from build123d import *

# Parameters (mm, degrees)
F3_DEPTH        = 1.651
F3_COPIES_COUNT = 10
F6_W            = 25.4
F6_H            = 5.08
F7_DEPTH        = 6.35
F8_R            = 1.5875
F9_DEPTH        = 3.81
F9_DEPTH_BACK   = 19.05
F10_R           = 9.906
F11_DEPTH       = 12.7
F12_R           = 9.525
F13_DEPTH       = 57.15
F14_R           = 7.62
F15_DEPTH       = 44.45


# Not quite as in the source:
# - a feature of the source that left no trace in its solid (it failed there, or was rolled back) is left out
# - a pattern or mirror of a feature is missing from the dataset's text; its kind, count and spacing are read off the source's solid


with BuildPart() as f1:
    # F0 (on Front) → F1 (revolve)
    with BuildSketch(Plane.XZ):
        with BuildLine():
            Line((-43.18, 1.016), (-45.6726494673, 1.016))
            ThreePointArc((-45.6726494673, 1.016), (-44.3886326409, 15.9499637645), (-57.15, 23.8125))
            Line((-57.15, 23.8125), (-57.15, -0.0228488987))
            Line((-57.15, -0.0228488987), (-43.18, -0.0228488987))
            Line((-43.18, -0.0228488987), (-43.18, 1.016))
        make_face()
    revolve(axis=Axis((-57.15, 0, 11.8948255506), (0, 0, 1)))

    # F2 (on face) → F3 (join)
    with BuildSketch(Plane.XY.offset(1.016)):
        with BuildLine():
            ThreePointArc((-45.6726494673, 0), (-45.6729398633, -0.081644771), (-45.6738110366, -0.1632854104))
            Line((-45.6738110366, -0.1632854104), (-43.1842536235, -0.1632854104))
            Line((-43.1842536235, -0.1632854104), (-43.1842536235, 0.3447145896))
            Line((-43.1842536235, 0.3447145896), (-45.6738110366, 0.3447145896))
            Line((-45.6738110366, 0.3447145896), (-45.6738110366, 0.1632854104))
            ThreePointArc((-45.6738110366, 0.1632854104), (-45.6729398633, 0.081644771), (-45.6726494673, 0))
        make_face()
    f3 = extrude(amount=F3_DEPTH)

    # F3_copies: F3 ×10 about axis
    f3_copies_axis = Axis((-57.15, 0, 0), (0, 0, 1))
    for i in range(1, F3_COPIES_COUNT):
        add(f3.rotate(f3_copies_axis, i * 360 / F3_COPIES_COUNT))

    # F6 (on offset) → F7 (cut)
    with BuildSketch(Plane.XY.offset(16.51)):
        with Locations((-57.15, 10.16)):
            Rectangle(F6_W, F6_H)
        with Locations((-57.15, -10.16)):
            Rectangle(F6_W, F6_H)
    extrude(amount=F7_DEPTH, mode=Mode.SUBTRACT)

    # F8 (on face) → F9 (cut, two sides)
    with BuildSketch(Plane.XZ.offset(7.62)) as f9_sk:
        with Locations((-57.15, 19.05)):
            Circle(F8_R)
    extrude(amount=F9_DEPTH, mode=Mode.SUBTRACT)
    extrude(f9_sk.sketch, amount=-F9_DEPTH_BACK, mode=Mode.SUBTRACT)

    # F10 (on face) → F11 (cut)
    with BuildSketch(Plane(origin=(0, 0, -0.0228488987), x_dir=(1, 0, 0), z_dir=(0, 0, -1))):
        with Locations((-57.15, 0)):
            Circle(F10_R)
    extrude(amount=-F11_DEPTH, mode=Mode.SUBTRACT)


with BuildPart() as f13:
    # F12 (on Top) → F13 (new body)
    with BuildSketch(Plane.XY):
        Circle(F12_R)
    extrude(amount=F13_DEPTH)

    # F14 (on face) → F15 (cut)
    with BuildSketch(Plane(origin=(0, 0, 0), x_dir=(1, 0, 0), z_dir=(0, 0, -1))):
        Circle(F14_R)
    extrude(amount=-F15_DEPTH, mode=Mode.SUBTRACT)


solid = f1.part
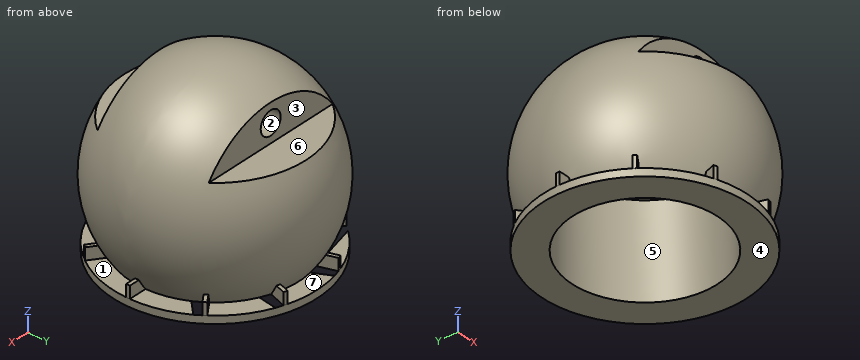
Input: part model. Units: mm. Frame: model coordinates. Face numbers are marked on the shaded views. A direction names the side the tool comes from. Give positions to 0.01 mm unless a question says otherwise; leave off trailing zeros. Write each loop counter-clockwise with the first axis right and the second up, starting at its lowest first coordinate (ties: lowest second). Pieces come first, ordered by that corner, then holes. Notation, with made-up numbers: M 11,-38 L 15,-38 A30 ccw 15,-12 Z; hole C -15.75,77 d9. An arc over 180 degrees is marked long. Use one line per item in the form item = value.
1. Cut plane B-B on x = -57.15. Return loops of the section in (y, z) (1 decimal).
Outcome:
outline = M -14,0 L -9.9,0 L -9.9,12.7 L 9.9,12.7 L 9.9,0 L 14,0 L 14,1 L 11.5,1 A14.3 ccw 12.5,16.5 L 7.6,16.5 L 7.6,17.5 L -7.6,17.5 L -7.6,16.5 L -12.5,16.5 A14.3 ccw -11.5,1 L -14,1 Z; M -7.6,20.6 L 7.6,20.6 L 7.6,21.6 A14.3 ccw -7.6,21.6 Z
2. First-contact query: P1, Ø2, axis at x = -54, y = -5.5, coming from the -Z side; P2, Ø0.7, axis at x = -53, y = -12.5, coming from the +Z side; P3, Ø3, axis at y = 4.5, z = 3, coming from the -X side. Flat tips, straight axial feed; report the tip coordinate or a pass-through.
Outcome:
P1 = 12.68
P2 = 15.83
P3 = -69.91
3. Cut plane D-D on x = -51.5. Return loops of the section in (y, z) (3 decimals).
Outcome:
outline = M -12.776,-0.023 L -8.137,-0.023 L -8.137,12.677 L 8.137,12.677 L 8.137,-0.023 L 12.776,-0.023 L 12.776,1.016 L 9.99,1.016 A13.123 ccw 11.109,16.51 L 7.62,16.51 L 7.62,20.209 A13.123 ccw -7.62,20.209 L -7.62,16.51 L -11.109,16.51 A13.123 ccw -9.99,1.016 L -12.776,1.016 Z
4. Mould query, pull axis Y, two halves, no side actions, for the marked faces 1, 2 and 3. Classes: released by +Y, released by -Y, zero draft, split by the parting line, or undercut.
Outcome:
face_1 = undercut
face_2 = zero draft
face_3 = released by +Y
5. Cut plane A-A on z = 19.05. Return loops of the section in (x, y).
Outcome:
outline = M -64.59,-7.62 L -58.74,-7.62 L -58.74,7.62 L -64.59,7.62 A10.65 ccw Z; M -55.56,-7.62 L -49.71,-7.62 A10.65 ccw -49.71,7.62 L -55.56,7.62 Z
6. Ray query, L1, parallel to Z at x = -54.5, y = -10.25; L2, parallel to X at y = 0, z = 9.75; L3, parallel to X at y = 0, z = 4.5. Return the intervals inside material, ascending.
Outcome:
L1 = -0.02 to 16.51
L2 = -71.44 to -67.06, -47.24 to -42.86
L3 = -70.52 to -67.06, -47.24 to -43.78
7. Reachability of the marked faces 4, 5, 6 and 7 from +Z, -Z, +X, -X, +Y, -Y: full face, straight path, thin tool, end or side. Return the list, or none.
Outcome:
face_4 = -Z, +X, -X, +Y, -Y
face_5 = -Z
face_6 = +Z, +X, -X, +Y
face_7 = +Y
